The model under review builds one solid part; all positions refer to its coordinate system, in mm. A direction names the side the tool comes from. Round coordinates to 2 decimals unless told otherwise and drop trailing zeros. Loops run counter-clockwise (first coordinate to the right, second up) from the corner with the lowest first, then second, coordinate; pieces in that order, holes last. Notation, with made-up numbers: M 12.25,52.25 L 62.25,52.25 A18 cw 62.25,87.25 Z; hole C 27.5,60 d11. An arc over 180 degrees is marked long. One line per question, with ' | ' between items.
from build123d import *

# Parameters (mm, degrees)
SKETCH_2_W      = 80
SKETCH_2_H      = 40
SKETCH_2_R      = 1.5
EXTRUDE_1_DEPTH = 1.5
SKETCH_3_R      = 3.3
SKETCH_3_R_2    = 1.5
EXTRUDE_2_DEPTH = 1


with BuildPart() as part:
    # 草图2 → 凸台-拉伸1 (new body)
    with BuildSketch(Plane.XY):
        with Locations((-7.229146383, 0.256789608)):
            Rectangle(SKETCH_2_W, SKETCH_2_H)
        with Locations((-22.479146383, 15.506789608)):
            Circle(SKETCH_2_R, mode=Mode.SUBTRACT)
        with Locations(Location((8.020853617, 15.506789608, 0), (0, 0, 180))):
            Circle(SKETCH_2_R, mode=Mode.SUBTRACT)
        with Locations((8.020853617, -14.993210392)):
            Circle(SKETCH_2_R, mode=Mode.SUBTRACT)
        with Locations(Location((-22.479146383, -14.993210392, 0), (0, 0, 180))):
            Circle(SKETCH_2_R, mode=Mode.SUBTRACT)
        Polygon((-7.229146383, -7.743210392), (0.770853617, -7.743210392), (0.770853617, 8.256789608), (-15.229146383, 8.256789608), (-15.229146383, -7.743210392), align=None, mode=Mode.SUBTRACT)
    extrude(amount=EXTRUDE_1_DEPTH)

    # 草图3 → 凸台-拉伸2 (add)
    # profile 1 of 4: a face of its own
    with BuildSketch(Plane.XY.offset(1.5)):
        with Locations((-22.479146383, 15.506789608)):
            Circle(SKETCH_3_R)
        with Locations((-22.479146383, 15.506789608)):
            Circle(SKETCH_3_R_2, mode=Mode.SUBTRACT)
    # profile 2 of 4: a face of its own
    with BuildSketch(Plane.XY.offset(1.5)):
        with Locations((8.020853617, 15.506789608)):
            Circle(SKETCH_3_R)
        with Locations(Location((8.020853617, 15.506789608, 0), (0, 0, 180))):
            Circle(SKETCH_3_R_2, mode=Mode.SUBTRACT)
    # profile 3 of 4: a face of its own
    with BuildSketch(Plane.XY.offset(1.5)):
        with Locations((-22.479146383, -14.993210392)):
            Circle(SKETCH_3_R)
        with Locations(Location((-22.479146383, -14.993210392, 0), (0, 0, 180))):
            Circle(SKETCH_3_R_2, mode=Mode.SUBTRACT)
    # profile 4 of 4: a face of its own
    with BuildSketch(Plane.XY.offset(1.5)):
        with Locations((8.020853617, -14.993210392)):
            Circle(SKETCH_3_R)
        with Locations((8.020853617, -14.993210392)):
            Circle(SKETCH_3_R_2, mode=Mode.SUBTRACT)
    extrude(amount=EXTRUDE_2_DEPTH)


solid = part.part
1) Add section B-B on x = -11.5. State the section outline as (y, z) points.
Output values:
outline: M -19.74,0 L -7.74,0 L -7.74,1.5 L -19.74,1.5 Z; M 8.26,0 L 20.26,0 L 20.26,1.5 L 8.26,1.5 Z
2) Add section C-C on z = 0.5. State the section outline as (x, y) points.
Output values:
outline: M -47.23,-19.74 L 32.77,-19.74 L 32.77,20.26 L -47.23,20.26 Z; hole C -22.48,-14.99 d3; hole C -22.48,15.51 d3; hole M -15.23,-7.74 L 0.77,-7.74 L 0.77,8.26 L -15.23,8.26 Z; hole C 8.02,-14.99 d3; hole C 8.02,15.51 d3
3) For line 1 (X direction, y = 15.5, z = 1.05); line 2 (X direction, y = 7.5, z = 0.55); line 3 (X direction, y = -15, z = 1.7), list the stretches that pass through material, from the lowest coordinate up.
Output values:
line 1: x = -47.23 to -23.98, -20.98 to 6.52, 9.52 to 32.77 | line 2: x = -47.23 to -15.23, 0.77 to 32.77 | line 3: x = -25.78 to -23.98, -20.98 to -19.18, 4.72 to 6.52, 9.52 to 11.32
4) Add section D-D on x = 10.5. State the section outline as (y, z) points, then the cut area to 3 significant figures.
Output values:
outline: M -19.74,0 L 20.26,0 L 20.26,1.5 L 17.68,1.5 L 17.68,2.5 L 13.33,2.5 L 13.33,1.5 L -12.82,1.5 L -12.82,2.5 L -17.17,2.5 L -17.17,1.5 L -19.74,1.5 Z | area: 68.7 mm²
5) Machinability: for faces 1 (the flat face through (-17, 1, 1.5)), 2 (the flat face through (0.771, 0, 1)), 3 (the flat face through (9, 14, 2.5)), which of the approach directions +Z, -Z, +X, -X, +Y, -Y give a long, thin tool a straight path to every point of the face, cutting with its end or side? Answer none if there is none.
Output values:
face 1: +Z | face 2: +Z, -Z | face 3: +Z, +X, -X, +Y, -Y
6) Mouldability with a two-part tool opening along X and no side actions: class faces 4 (the flat face through (-8, -19.743, 1)), 5 (the flat face through (-47.229, 0, 1)), 6 (the cylindrical face through (6.831, -15.906, 1.232)), 7 (the flat face through (32.771, 0, 1)) as +X half, -X half, draft (parallel to the pull), parting line (faces both ways), or undercut.
Output values:
face 4: draft | face 5: -X half | face 6: undercut | face 7: +X half
7) Insertion check: P1, Ø1, axis at x = 22.5, y = 0.5, coming from the +Z side. The pin has a flat end and moves straight along its axis. Give the tip position at first contact, or say it passes through.
Output values:
P1: stops at z = 1.5
8) Add section A-A on y = 7. State the section outline as (x, z) points, then the cut area to 3 significant figures.
Output values:
outline: M -47.23,0 L -15.23,0 L -15.23,1.5 L -47.23,1.5 Z; M 0.77,0 L 32.77,0 L 32.77,1.5 L 0.77,1.5 Z | area: 96.0 mm²
